The listing builds one solid part. Answer for the finished solid, in the listing's coordinates (mm). A direction names the side the tool comes from. Round coordinates to 2 decimals unless told otherwise and drop trailing zeros. Write each loop counter-clockwise with the first axis right and the second up, starting at its lowest first coordinate (ties: lowest second). Pieces come first, ordered by that corner, then holes.
Item 1: Find section A-A on z = 67. Give the vertices of the cut face in (x, y), then the cut area to 3 significant figures.
Item 2: A tool of negligible diameter and unlimited length cuts with its end or side. For faces 1 (the face through (14.654, -8.619, 116.409)), 2 (the face through (8, 8, 110)), from which of +Z, -Z, +X, -X, +Y, -Y can it reach the whole face along a straight path? Write none if from no direction.
Item 3: Each of these flat-tipped pins is pushed along its axis until it touches: pin 1 (4 mm diameter, centred on x = -5.5, z = 31, fed in from +Y); pin 2 (12 mm diameter, centred on y = 12, z = 66, fed in from -X); pin 3 (5 mm diameter, centred on y = 5, z = -11, fed in from +X). Where does it stop, or does it pass through?
Item 4: Find the intervals of material crossed by probe 1 along Y at (x, z) = (-2, -59); probe 2 along Z at (x, y) = (-9.5, -13), in increasing order.
```python
from build123d import *

# Parameters (mm, degrees)
SKETCH1_R           = 10
BOSS_EXTRUDE1_DEPTH = 110
BOSS_EXTRUDE2_DEPTH = 13
SKETCH3_OUTSIDE_W   = 134.036
SKETCH3_OUTSIDE_H   = 128.776
SKETCH3_OUTSIDE_R   = 17
CUT_EXTRUDE1_DEPTH  = 13
CUT_EXTRUDE1_DRAFT  = -60


with BuildPart() as part:
    # Sketch1 → Boss-Extrude1 (new, symmetric)
    with BuildSketch(Plane.XY):
        Circle(SKETCH1_R)
    extrude(amount=BOSS_EXTRUDE1_DEPTH, both=True)

    # Sketch2 → Boss-Extrude2 (add)
    with BuildSketch(Plane.XY.offset(110)):
        Polygon((-19.629909152, 0), (-9.814954576, -17), (9.814954576, -17), (19.629909152, 0), (9.814954576, 17), (-9.814954576, 17), align=None)
    extrude(amount=BOSS_EXTRUDE2_DEPTH)


with BuildPart() as cut_extrude1_tool:
    # Sketch3 outside → Cut-Extrude1 (with draft: the straight prism first)
    with BuildSketch(Plane.XY.offset(123)):
        Rectangle(SKETCH3_OUTSIDE_W, SKETCH3_OUTSIDE_H)
        Circle(SKETCH3_OUTSIDE_R, mode=Mode.SUBTRACT)
    extrude(amount=-CUT_EXTRUDE1_DEPTH)
    # Cut-Extrude1: the draft: its side faces are tilted about the plane it starts from
    cut_extrude1_sides = [cut_extrude1_tool.faces().sort_by_distance(p)[0] for p in [
        (0, -64.388, 116.5),
        (67.018, 0, 116.5),
        (0, 64.388, 116.5),
        (-67.018, 0, 116.5),
        (-17, 0, 116.5),
    ]]
    draft(cut_extrude1_sides, Plane.XY.offset(123), CUT_EXTRUDE1_DRAFT)


with BuildPart() as part_1:
    add(part.part)

    # Cut-Extrude1: cut by cut_extrude1_tool
    add(cut_extrude1_tool.part, mode=Mode.SUBTRACT)


solid = part_1.part
```
Check values:
1. outline: circle Ø20 at (0, 0)
1. area: 314 mm2
2. face 1: +Z, -Z, +X, -Y
2. face 2: -Z
3. pin 1: stops at y = 9.37
3. pin 2: stops at x = -8
3. pin 3: stops at x = 9.68
4. probe 1: y = -9.8 to 9.8
4. probe 2: z = 110 to 123
